Read the model definition and answer for the solid it produces. Units are mm, in the model's axes. A direction names the side the tool comes from. Give positions to 0.01 mm unless a question says otherwise; leave off trailing zeros. Loops run counter-clockwise (first coordinate to the right, second up) from the corner with the lowest first, then second, coordinate; pieces in that order, holes last. Notation, with made-up numbers: (69.5, 72) -> (76.5, 72) arc R18 ccw to (76.5, 91) -> close; hole circle Ø6 at (59.5, -11). An arc over 180 degrees is marked (long way). Return JSON: item names as keys, results as strings. Group by question number.
from build123d import *

# Parameters (mm, degrees)
EXTRUDE136140_DEPTH = 5
BOX017_W            = 41
BOX017_H            = 140
BOX017_DEPTH        = 60
SKETCH348_R         = 1.85
EXTRUDE136129_DEPTH = 25
EXTRUDE136133_DEPTH = 6
EXTRUDE136132_DEPTH = 6
SKETCH339_R         = 1.75
EXTRUDE136134_DEPTH = 14
EXTRUDE136135_DEPTH = 5
SKETCH349_R         = 2.85
EXTRUDE136130_DEPTH = 25
SKETCH353_R         = 2.75
EXTRUDE136137_DEPTH = 4
EXTRUDE136131_DEPTH = 116
EXTRUDE136138_DEPTH = 20.5
EXTRUDE136128_DEPTH = 8
EXTRUDE136127_DEPTH = 8
ARRAY032_COUNT      = 2
EXTRUDE136139_DEPTH = 5


with BuildPart() as extrude136140:
    # Sketch355 → Extrude136140 (new body)
    with BuildSketch(Plane.XZ):
        Polygon((0, 0), (-2, 0), (-3.443376, 2.5), (-3.443376, 9), (5.556624, 9), (5.556624, 2.5), (1.443376, 2.5), align=None)
    extrude(amount=-EXTRUDE136140_DEPTH)


with BuildPart() as extrude136140_1:
    # Extrude136140 placement: moved
    add(extrude136140.part.moved(Location((48, 42.5, -44))))


with BuildPart() as cube014:
    # Box017 → Box017 (new body)
    with BuildSketch(Plane(origin=(52, -70, -46), x_dir=(1, 0, 0), z_dir=(0, 0, 1))):
        with Locations((20.5, 70)):
            Rectangle(BOX017_W, BOX017_H)
    extrude(amount=BOX017_DEPTH)


with BuildPart() as extrude136129:
    # Sketch348 → Extrude136129 (new body)
    with BuildSketch(Plane.XY):
        with Locations((-40, 60)):
            Circle(SKETCH348_R)
        with Locations((40, 60)):
            Circle(SKETCH348_R)
        with Locations((40, -60)):
            Circle(SKETCH348_R)
        with Locations((-40, -60)):
            Circle(SKETCH348_R)
    extrude(amount=-EXTRUDE136129_DEPTH)


with BuildPart() as extrude136133:
    # Sketch351 → Extrude136133 (new body)
    with BuildSketch(Plane.XZ):
        Polygon((-4.05083, 4), (-1.25, 0), (1.25, 0), (4.05083, 4), align=None)
    extrude(amount=-EXTRUDE136133_DEPTH)


with BuildPart() as extrude136133_1:
    # Extrude136133 placement: moved
    add(extrude136133.part.moved(Location((0, 42, 0))))


with BuildPart() as fusion034004041077001011012:
    # Sketch351 → Extrude136132 (new body)
    with BuildSketch(Plane.XZ):
        Polygon((-4.05083, 4), (-1.25, 0), (1.25, 0), (4.05083, 4), align=None)
    extrude(amount=-EXTRUDE136132_DEPTH)


with BuildPart() as fusion034004041077001011012_1:
    # Extrude136132 placement: moved
    add(fusion034004041077001011012.part.moved(Location((0, -48, 0))))

    # Fusion034004041077001011012: union Extrude136133
    add(extrude136133_1.part)


with BuildPart() as fusion034004041077001011012_2:
    # Fusion034004041077001011012 placement: moved
    add(fusion034004041077001011012_1.part.moved(Location((47, 0, -44))))


with BuildPart() as extrude136134:
    # Sketch339 → Extrude136134 (new body)
    with BuildSketch(Plane.XY.offset(-32)):
        with Locations((-37.5, 46.5)):
            Circle(SKETCH339_R)
        with Locations((37.5, 46.5)):
            Circle(SKETCH339_R)
        with Locations((37.5, -46.5)):
            Circle(SKETCH339_R)
        with Locations((-37.5, -46.5)):
            Circle(SKETCH339_R)
    extrude(amount=-EXTRUDE136134_DEPTH)


with BuildPart() as extrude136135:
    # Sketch340 → Extrude136135 (new body)
    with BuildSketch(Plane.XY.offset(-39)):
        Polygon((39.125, -49.314583), (40.75, -46.5), (39.125, -43.685417), (35.875, -43.685417), (34.25, -46.5), (35.875, -49.314583), align=None)
        Polygon((39.125, 43.685417), (40.75, 46.5), (39.125, 49.314583), (35.875, 49.314583), (34.25, 46.5), (35.875, 43.685417), align=None)
        Polygon((-34.25, 46.5), (-35.875, 49.314583), (-39.125, 49.314583), (-40.75, 46.5), (-39.125, 43.685417), (-35.875, 43.685417), align=None)
        Polygon((-40.75, -46.5), (-39.125, -49.314583), (-35.875, -49.314583), (-34.25, -46.5), (-35.875, -43.685417), (-39.125, -43.685417), align=None)
    extrude(amount=EXTRUDE136135_DEPTH)


with BuildPart() as fusion034004041077001011011:
    # Sketch349 → Extrude136130 (new body)
    with BuildSketch(Plane.XY.offset(-8)):
        with Locations((-40, -60)):
            Circle(SKETCH349_R)
        with Locations((40, -60)):
            Circle(SKETCH349_R)
        with Locations((40, 60)):
            Circle(SKETCH349_R)
        with Locations((-40, 60)):
            Circle(SKETCH349_R)
    extrude(amount=-EXTRUDE136130_DEPTH)

    # Fusion034004041077001011011: union Extrude136129, Fusion034004041077001011012, Extrude136134, Extrude136135
    add(extrude136129.part)
    add(fusion034004041077001011012_2.part)
    add(extrude136134.part)
    add(extrude136135.part)


with BuildPart() as loft005:
    # Sketch344 → Loft005 section 0
    with BuildSketch(Plane.XY.offset(-42)):
        with BuildLine():
            Line((83.953856, 28), (74.656255, 47.938771))
            Line((-74.656255, 47.938771), (74.656255, 47.938771))
            Line((-74.656255, 47.938771), (-83.953856, 28))
            ThreePointArc((-83.953856, -28), (-79.195376, 0), (-83.953856, 28))
            Line((-83.953856, -28), (-74.656255, -47.938771))
            Line((-74.656255, -47.938771), (74.656255, -47.938771))
            Line((74.656255, -47.938771), (83.953856, -28))
            ThreePointArc((83.953856, 28), (79.195376, 0), (83.953856, -28))
        make_face()
    # Sketch345 → Loft005 section 1
    with BuildSketch(Plane.XY.offset(-5)):
        with BuildLine():
            Line((86.49793, 28.2685), (67.99793, 60.31144))
            Line((-67.99793, 60.31144), (67.99793, 60.31144))
            Line((-67.99793, 60.31144), (-86.49793, 28.2685))
            ThreePointArc((-86.49793, -28.2685), (-78.355592, 0), (-86.49793, 28.2685))
            Line((-86.49793, -28.2685), (-67.99793, -60.31144))
            Line((-67.99793, -60.31144), (67.99793, -60.31144))
            Line((67.99793, -60.31144), (86.49793, -28.2685))
            ThreePointArc((86.49793, 28.2685), (78.355592, 0), (86.49793, -28.2685))
        make_face()
    # Sketch343 → Loft005 section 2
    with BuildSketch(Plane.XY.offset(12)):
        with BuildLine():
            Line((86.49793, 28.2685), (67.99793, 60.31144))
            Line((-67.99793, 60.31144), (67.99793, 60.31144))
            Line((-67.99793, 60.31144), (-86.49793, 28.2685))
            ThreePointArc((-86.49793, -28.2685), (-78.355592, 0), (-86.49793, 28.2685))
            Line((-86.49793, -28.2685), (-67.99793, -60.31144))
            Line((-67.99793, -60.31144), (67.99793, -60.31144))
            Line((67.99793, -60.31144), (86.49793, -28.2685))
            ThreePointArc((86.49793, 28.2685), (78.355592, 0), (86.49793, -28.2685))
        make_face()
    loft(ruled=True)


with BuildPart() as extrude136137:
    # Sketch353 → Extrude136137 (new body)
    with BuildSketch(Plane.YZ):
        Polygon((-6.25, 0), (-6.25, 7.75), (-2.5, 11.5), (2.5, 11.5), (6.25, 7.75), (6.25, 0), align=None)
        with Locations((0, 6.5)):
            Circle(SKETCH353_R, mode=Mode.SUBTRACT)
    extrude(amount=EXTRUDE136137_DEPTH)


with BuildPart() as extrude136137_1:
    # Extrude136137 placement: moved
    add(extrude136137.part.moved(Location((78, 0, 0))))


with BuildPart() as cut009010006006006005025006:
    # Sketch342 → Loft006 section 0
    with BuildSketch(Plane.XY.offset(-44)):
        with BuildLine():
            Line((86.585218, 28), (76.019762, 50.657695))
            Line((-76.019762, 50.657695), (76.019762, 50.657695))
            Line((-76.019762, 50.657695), (-86.585218, 28))
            ThreePointArc((-86.585218, -28), (-81.826738, 0), (-86.585218, 28))
            Line((-86.585218, -28), (-76.019762, -50.657695))
            Line((-76.019762, -50.657695), (76.019762, -50.657695))
            Line((76.019762, -50.657695), (86.585218, -28))
            ThreePointArc((86.585218, 28), (81.826738, 0), (86.585218, -28))
        make_face()
    # Sketch346 → Loft006 section 1
    with BuildSketch(Plane.XY.offset(-5)):
        with BuildLine():
            Line((89.648714, 28.2685), (69.148714, 63.775542))
            Line((-69.148714, 63.775542), (69.148714, 63.775542))
            Line((-69.148714, 63.775542), (-89.648714, 28.2685))
            ThreePointArc((-89.648714, -28.2685), (-81.506376, 0), (-89.648714, 28.2685))
            Line((-89.648714, -28.2685), (-69.148714, -63.775542))
            Line((-69.148714, -63.775542), (69.148714, -63.775542))
            Line((69.148714, -63.775542), (89.648714, -28.2685))
            ThreePointArc((89.648714, 28.2685), (81.506376, 0), (89.648714, -28.2685))
        make_face()
    # Sketch341 → Loft006 section 2
    with BuildSketch(Plane.XY):
        with BuildLine():
            Line((89.648714, 28.2685), (69.148714, 63.775542))
            Line((-69.148714, 63.775542), (69.148714, 63.775542))
            Line((-69.148714, 63.775542), (-89.648714, 28.2685))
            ThreePointArc((-89.648714, -28.2685), (-81.506376, 0), (-89.648714, 28.2685))
            Line((-89.648714, -28.2685), (-69.148714, -63.775542))
            Line((-69.148714, -63.775542), (69.148714, -63.775542))
            Line((69.148714, -63.775542), (89.648714, -28.2685))
            ThreePointArc((89.648714, 28.2685), (81.506376, 0), (89.648714, -28.2685))
        make_face()
    loft(ruled=True)

    # Fusion034004041077001011013: union Extrude136137
    add(extrude136137_1.part)

    # Cut009010006006006005025006: cut Loft005
    add(loft005.part, mode=Mode.SUBTRACT)


with BuildPart() as extrude136131:
    # Sketch350 → Extrude136131 (new body)
    with BuildSketch(Plane.YZ):
        Polygon((-52.764154, 0), (-49.5, -7), (-42.5, -7), (-42.5, 0), align=None)
        Polygon((52.764154, 0), (49.5, -7), (42.5, -7), (42.5, 0), align=None)
        Polygon((-26, 0), (-23, 0), (-23, -7), (-30.041452, -7), align=None)
        Polygon((23, 0), (26, 0), (30.041452, -7), (23, -7), align=None)
    extrude(amount=EXTRUDE136131_DEPTH)


with BuildPart() as extrude136131_1:
    # Extrude136131 placement: moved
    add(extrude136131.part.moved(Location((-72.85, 0, -35))))


with BuildPart() as extrude136138:
    # Sketch354 → Extrude136138 (new body)
    with BuildSketch(Plane.YZ):
        Polygon((-52.764154, 0), (-49.5, -7), (-42.5, -7), (-42.5, 0), align=None)
        Polygon((52.764154, 0), (49.5, -7), (42.5, -7), (42.5, 0), align=None)
    extrude(amount=-EXTRUDE136138_DEPTH)


with BuildPart() as extrude136138_1:
    # Extrude136138 placement: moved
    add(extrude136138.part.moved(Location((72.75, 0, -35))))


with BuildPart() as extrude136128:
    # Sketch347 → Extrude136128 (new body)
    with BuildSketch(Plane.YZ):
        Polygon((0, 0), (0, -5), (7, -17.124356), (7, 0), align=None)
    extrude(amount=EXTRUDE136128_DEPTH)


with BuildPart() as extrude136128_1:
    # Extrude136128 placement: moved
    add(extrude136128.part.moved(Location((-44, -63, 0))))


with BuildPart() as common001:
    # Sketch347 → Extrude136127 (new body)
    with BuildSketch(Plane.YZ):
        Polygon((0, 0), (0, -5), (7, -17.124356), (7, 0), align=None)
    extrude(amount=EXTRUDE136127_DEPTH)


with BuildPart() as common001_1:
    # Extrude136127 placement: moved
    add(common001.part.moved(Location((36, -63, 0))))

    # Fusion034004041077001011010: union Extrude136128
    add(extrude136128_1.part)

    # Array032: Common001 ×2 about axis
    array032_axis = Axis((0, 0, 0), (0, 0, 1))


with BuildPart() as common001_2:
    add(common001_1.part)
    for i in range(1, ARRAY032_COUNT):
        add(common001_1.part.rotate(array032_axis, i * 360 / ARRAY032_COUNT))

    # Fusion034004041077001011014: union Cut009010006006006005025006, Extrude136131, Extrude136138
    add(cut009010006006006005025006.part)
    add(extrude136131_1.part)
    add(extrude136138_1.part)

    # Cut009010006006006005025007: cut Fusion034004041077001011011
    add(fusion034004041077001011011.part, mode=Mode.SUBTRACT)

    # Common001: intersect Cube014
    add(cube014.part, mode=Mode.INTERSECT)


with BuildPart() as batterycoverfusion44mm:
    # Sketch355 → Extrude136139 (new body)
    with BuildSketch(Plane.XZ):
        Polygon((0, 0), (-2, 0), (-3.443376, 2.5), (-3.443376, 9), (5.556624, 9), (5.556624, 2.5), (1.443376, 2.5), align=None)
    extrude(amount=EXTRUDE136139_DEPTH)


with BuildPart() as batterycoverfusion44mm_1:
    # Extrude136139 placement: moved
    add(batterycoverfusion44mm.part.moved(Location((48, -42.5, -44))))

    # Fusion034004041077001011015: union Extrude136140, Common001
    add(extrude136140_1.part)
    add(common001_2.part)


with BuildPart() as batterycoverfusion44mm_2:
    # Fusion034004041077001011015 placement: moved
    add(batterycoverfusion44mm_1.part.moved(Location((0, 0, -25.5))))


solid = batterycoverfusion44mm_2.part
1. Straight lines are drawn through the part: line 1 (Z direction, x = 79.3, y = 0); line 2 (Y direction, x = 80, z = -19); line 3 (Y direction, x = 52.5, z = -27). For each, find the intervals that lie inside material, in ascending order. Write a range as from..to.
2. Which of the six approach directions +Z, -Z, +X, -X, +Y, -Y give full straight-line access (tool end or side, diameter ignored) to faces 1 (the flat face through (45.29, -44.96, -68.27)), 2 (the cylindrical face through (78.357, -0.417, -25.801)), 3 (the flat face through (72.75, 46, -64)), 4 (the flat face through (80, -6.25, -22)), 5 (the flat face through (48.732, -44.965, -68.232))?
3. Determine the mould class of faces 6 (the flat face through (77.377, 44.066, -27.965)), 7 (the cylindrical face through (81.51, -0.42, -27.96)), 8 (the flat face through (80, 0, -14)) for opening direction Z: pulls with the +Z half, pulls with the -Z half, needs draft (parallel to the pull), parting line crosses it, or undercut.
4. Flat-ended cylindrical pins translate along their axes: pin 1 Ø9 at (y, z) = (0, -19) entering from +X; pin 2 Ø4.5 at (x, z) = (58.5, -67) entering from +Y; pin 3 Ø10 at (y, z) = (11, -50) entering from -X. Find the tip coordinate at first contact, or state that the pin passes through.
5. Section A-A on z = -19 is taken. Determine the outline of the cut face in (x, y), then the cut area to 3 significant figures.
Completed:
{
 "1": {"line 1": "z = -69.5..-21.75, -16.25..-14", "line 2": "y = -6.25..-2.75, 2.75..6.25", "line 3": "y = -63.78..-60.31, 60.31..63.78"},
 "2": {"face 1": "-Z, -X, +Y, -Y", "face 2": "+Z, -X", "face 3": "+Z", "face 4": "+Z, +X, -X, -Y", "face 5": "-Z, +Y, -Y"},
 "3": {"face 6": "needs draft", "face 7": "undercut", "face 8": "pulls with the +Z half"},
 "4": {"pin 1": "stops at x = 82", "pin 2": "stops at y = 52.26", "pin 3": "stops at x = 79.06"},
 "5": {"outline": "(78.43, -2.75) arc R53.14 ccw to (78.72, -6.25) -> (82, -6.25) -> (82, -2.75) -> close; (78.43, 2.75) -> (82, 2.75) -> (82, 6.25) -> (78.72, 6.25) arc R53.14 ccw to start", "area": "24.1 mm²"}
}
